Could you check a few things on this model? Use its own coordinates, in mm. Face numbers are marked on the shaded views. A direction names the side the tool comes from. Give positions to 0.01 mm unless a question says otherwise; leave off trailing zeros. Loops run counter-clockwise (first coordinate to the right, second up) from the corner with the lowest first, then second, coordinate; pieces in that order, holes last.
1. Imagine slicing it at B-B (z = -17.5). List the corners of the cut face in (x, y) for me.
2. I need wall thicknesses on line 1 along X through (y, z) = (24, -5.5); line 2 along Y through (x, z) = (71.5, -3.25). Which ranges of each line are inside material? Lowest first, please.
3. For the marked faces 1 and 2, which set-ups out of +Z, -Z, +X, -X, +Y, -Y let a thin tool reach every point of the face, with its end or its side?
4. Imagine slicing it at C-C (x = 54). List the corners of the cut face in (y, z) for me.
5. Imagine slicing it at A-A (y = 18). List the corners of the cut face in (x, z) for me.
6. Thinking about a two-plate mould opening in X: for the marked faces 3, 4 and 5, which applies, +X half, -X half, draft (parallel to the pull), parting line (faces both ways), or undercut?
7. For P1, Ø6, axis at x = 170, z = -9.5, coming from the +Y side, with a flat end and sliding along its axis, tell me the tip position at first contact or that it passes through.
```python
from build123d import *

# Parameters (mm, degrees)
SKETCH_1_W                       = 301
SKETCH_1_H                       = 20
SM_BASE_FLANGE_1_DEPTH           = 1.5
SM_EDGE_FLANGE_1_STRIP_W         = 7.4732
SM_EDGE_FLANGE_1_STRIP_H         = 1.5
SM_EDGE_FLANGE_1_STRIP_CUT_DEPTH = 20
SM_EDGE_FLANGE_1_DEPTH           = 20
SM_EDGE_FLANGE_2_STRIP_W         = 7.4732
SM_EDGE_FLANGE_2_STRIP_H         = 1.5
SM_EDGE_FLANGE_2_STRIP_CUT_DEPTH = 20
SM_EDGE_FLANGE_2_DEPTH           = 20


# Sheet-metal steps are written as plain solids
with BuildPart() as part:
    # Sketch 1 → Базовая кромка1 (new body)
    with BuildSketch(Plane(origin=(0, 0, 0), x_dir=(1, 0, 0), z_dir=(0, 1, 0))):
        with Locations((150.5, 10)):
            Rectangle(SKETCH_1_W, SKETCH_1_H)
    extrude(amount=-SM_BASE_FLANGE_1_DEPTH)

    # Ребро-кромка1 strip (across the edge) → Ребро-кромка1 strip cut (cut)
    with BuildSketch(Plane.XY.offset(-20)):
        with Locations((-1.5, -0.75)):
            Rectangle(SM_EDGE_FLANGE_1_STRIP_W, SM_EDGE_FLANGE_1_STRIP_H)
    extrude(amount=SM_EDGE_FLANGE_1_STRIP_CUT_DEPTH, mode=Mode.SUBTRACT)

    # Ребро-кромка1 section (across the edge) → Ребро-кромка1 (add)
    with BuildSketch(Plane.XY.offset(-20)):
        with BuildLine():
            Line((0, 0.7366), (0, 33.5))
            Line((0, 33.5), (1.5, 33.5))
            Line((1.5, 33.5), (1.5, 0.7366))
            ThreePointArc((1.5, 0.7366), (1.715745145, 0.215745145), (2.2366, 0))
            Line((2.2366, 0), (2.2366, -1.5))
            ThreePointArc((2.2366, -1.5), (0.655084973, -0.844915027), (0, 0.7366))
        make_face()
    extrude(amount=SM_EDGE_FLANGE_1_DEPTH)

    # Ребро-кромка2 strip (across the edge) → Ребро-кромка2 strip cut (cut)
    with BuildSketch(Plane(origin=(301, 0, 0), x_dir=(-1, 0, 0), z_dir=(0, 0, -1))):
        with Locations((-1.5, -0.75)):
            Rectangle(SM_EDGE_FLANGE_2_STRIP_W, SM_EDGE_FLANGE_2_STRIP_H)
    extrude(amount=SM_EDGE_FLANGE_2_STRIP_CUT_DEPTH, mode=Mode.SUBTRACT)

    # Ребро-кромка2 section (across the edge) → Ребро-кромка2 (add)
    with BuildSketch(Plane(origin=(301, 0, 0), x_dir=(-1, 0, 0), z_dir=(0, 0, -1))):
        with BuildLine():
            Line((0, 0.7366), (0, 33.5))
            Line((0, 33.5), (1.5, 33.5))
            Line((1.5, 33.5), (1.5, 0.7366))
            ThreePointArc((1.5, 0.7366), (1.715745145, 0.215745145), (2.2366, 0))
            Line((2.2366, 0), (2.2366, -1.5))
            ThreePointArc((2.2366, -1.5), (0.655084973, -0.844915027), (0, 0.7366))
        make_face()
    extrude(amount=SM_EDGE_FLANGE_2_DEPTH)


solid = part.part
```
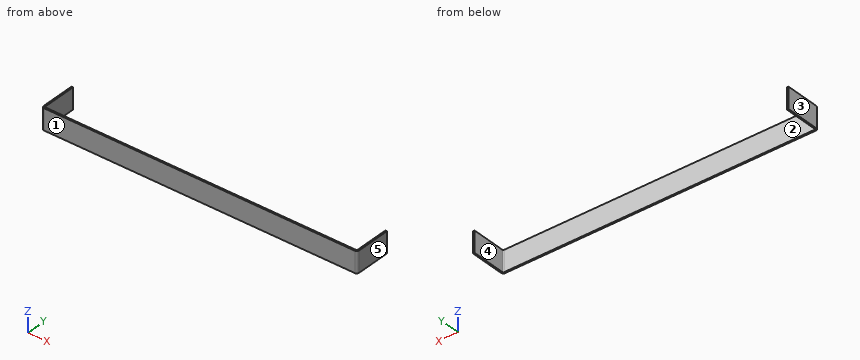
Derived:
1. outline: (0, 0.74) arc R2.24 ccw to (2.24, -1.5) - (298.76, -1.5) arc R2.24 ccw to (301, 0.74) - (301, 33.5) - (299.5, 33.5) - (299.5, 0.74) arc R0.74 cw to (298.76, 0) - (2.24, 0) arc R0.74 cw to (1.5, 0.74) - (1.5, 33.5) - (0, 33.5) - close
2. line 1: x = 0 to 1.5, 299.5 to 301
2. line 2: y = -1.5 to 0
3. face 1: +Z, -Z, +X, -X, -Y
3. face 2: +Z, -Z, +Y
4. outline: (-1.5, -20) - (0, -20) - (0, 0) - (-1.5, 0) - close
5. outline: (0, -20) - (1.5, -20) - (1.5, 0) - (0, 0) - close; (299.5, -20) - (301, -20) - (301, 0) - (299.5, 0) - close
6. face 3: -X half
6. face 4: undercut
6. face 5: +X half
7. P1: stops at y = 0
